from build123d import *

# Parameters (mm, degrees)
SKETCH1_W           = 16.51
SKETCH1_H           = 17.78
BOSS_EXTRUDE1_DEPTH = 1.778
FILLET1_R           = 2.54
CUT_EXTRUDE1_REACH  = 14.261
SKETCH2_R           = 0.508
SKETCH4_W           = 3.95
SKETCH4_H           = 3.95
BOSS_EXTRUDE3_DEPTH = 1.397
CUT_EXTRUDE2_REACH  = 14.261
SKETCH5_R           = 1.27


with BuildPart() as part:
    # Sketch1 → Boss-Extrude1 (new body)
    with BuildSketch(Plane(origin=(0, 0, 0), x_dir=(1, 0, 0), z_dir=(0, 1, 0))):
        Rectangle(SKETCH1_W, SKETCH1_H)
    extrude(amount=BOSS_EXTRUDE1_DEPTH)

    # Fillet1
    fillet1_edges = [part.edges().sort_by_distance(p)[0] for p in [
        (8.255, 0.889, 8.89),
        (-8.255, 0.889, 8.89),
        (-8.255, 0.889, -8.89),
        (8.255, 0.889, -8.89),
    ]]
    fillet(fillet1_edges, radius=FILLET1_R)

    # Sketch2 → Cut-Extrude1 (cut, up to next)
    with BuildSketch(Plane(origin=(0, 1.778, 0), x_dir=(1, 0, 0), z_dir=(0, 1, 0)), mode=Mode.PRIVATE) as cut_extrude1_sk1:
        with Locations(Location((-6.35, -7.112, 0), (0, 0, 270))):
            Circle(SKETCH2_R)
    cut_extrude1_tool1 = extrude(cut_extrude1_sk1.sketch, amount=-CUT_EXTRUDE1_REACH, mode=Mode.PRIVATE) & part.part
    # Sketch2 → Cut-Extrude1 (cut, up to next)
    with BuildSketch(Plane(origin=(0, 1.778, 0), x_dir=(1, 0, 0), z_dir=(0, 1, 0)), mode=Mode.PRIVATE) as cut_extrude1_sk2:
        with Locations(Location((-3.81, -7.112, 0), (0, 0, 270))):
            Circle(SKETCH2_R)
    cut_extrude1_tool2 = extrude(cut_extrude1_sk2.sketch, amount=-CUT_EXTRUDE1_REACH, mode=Mode.PRIVATE) & part.part
    # Sketch2 → Cut-Extrude1 (cut, up to next)
    with BuildSketch(Plane(origin=(0, 1.778, 0), x_dir=(1, 0, 0), z_dir=(0, 1, 0)), mode=Mode.PRIVATE) as cut_extrude1_sk3:
        with Locations(Location((-1.27, -7.112, 0), (0, 0, 270))):
            Circle(SKETCH2_R)
    cut_extrude1_tool3 = extrude(cut_extrude1_sk3.sketch, amount=-CUT_EXTRUDE1_REACH, mode=Mode.PRIVATE) & part.part
    # Sketch2 → Cut-Extrude1 (cut, up to next)
    with BuildSketch(Plane(origin=(0, 1.778, 0), x_dir=(1, 0, 0), z_dir=(0, 1, 0)), mode=Mode.PRIVATE) as cut_extrude1_sk4:
        with Locations(Location((1.27, -7.112, 0), (0, 0, 270))):
            Circle(SKETCH2_R)
    cut_extrude1_tool4 = extrude(cut_extrude1_sk4.sketch, amount=-CUT_EXTRUDE1_REACH, mode=Mode.PRIVATE) & part.part
    # Sketch2 → Cut-Extrude1 (cut, up to next)
    with BuildSketch(Plane(origin=(0, 1.778, 0), x_dir=(1, 0, 0), z_dir=(0, 1, 0)), mode=Mode.PRIVATE) as cut_extrude1_sk5:
        with Locations(Location((3.81, -7.112, 0), (0, 0, 270))):
            Circle(SKETCH2_R)
    cut_extrude1_tool5 = extrude(cut_extrude1_sk5.sketch, amount=-CUT_EXTRUDE1_REACH, mode=Mode.PRIVATE) & part.part
    # Sketch2 → Cut-Extrude1 (cut, up to next)
    with BuildSketch(Plane(origin=(0, 1.778, 0), x_dir=(1, 0, 0), z_dir=(0, 1, 0)), mode=Mode.PRIVATE) as cut_extrude1_sk6:
        with Locations(Location((6.35, -7.112, 0), (0, 0, 270))):
            Circle(SKETCH2_R)
    cut_extrude1_tool6 = extrude(cut_extrude1_sk6.sketch, amount=-CUT_EXTRUDE1_REACH, mode=Mode.PRIVATE) & part.part
    add(cut_extrude1_tool1.solids().sort_by_distance((-6.35, 1.778, 7.112))[0], mode=Mode.SUBTRACT)
    add(cut_extrude1_tool2.solids().sort_by_distance((-3.81, 1.778, 7.112))[0], mode=Mode.SUBTRACT)
    add(cut_extrude1_tool3.solids().sort_by_distance((-1.27, 1.778, 7.112))[0], mode=Mode.SUBTRACT)
    add(cut_extrude1_tool4.solids().sort_by_distance((1.27, 1.778, 7.112))[0], mode=Mode.SUBTRACT)
    add(cut_extrude1_tool5.solids().sort_by_distance((3.81, 1.778, 7.112))[0], mode=Mode.SUBTRACT)
    add(cut_extrude1_tool6.solids().sort_by_distance((6.35, 1.778, 7.112))[0], mode=Mode.SUBTRACT)

    # Sketch4 → Boss-Extrude3 (add)
    with BuildSketch(Plane(origin=(0, 0, 0), x_dir=(-1, 0, 0), z_dir=(0, -1, 0))):
        with Locations((0, 1.27)):
            Rectangle(SKETCH4_W, SKETCH4_H)
    extrude(amount=BOSS_EXTRUDE3_DEPTH)

    # Sketch5 → Cut-Extrude2 (cut, up to next)
    with BuildSketch(Plane(origin=(0, 0, 0), x_dir=(-1, 0, 0), z_dir=(0, -1, 0)), mode=Mode.PRIVATE) as cut_extrude2_sk1:
        with Locations(Location((-5.715, 6.35, 0), (0, 0, 90))):
            Circle(SKETCH5_R)
    cut_extrude2_tool1 = extrude(cut_extrude2_sk1.sketch, amount=-CUT_EXTRUDE2_REACH, mode=Mode.PRIVATE) & part.part
    # Sketch5 → Cut-Extrude2 (cut, up to next)
    with BuildSketch(Plane(origin=(0, 0, 0), x_dir=(-1, 0, 0), z_dir=(0, -1, 0)), mode=Mode.PRIVATE) as cut_extrude2_sk2:
        with Locations(Location((5.715, 6.35, 0), (0, 0, 90))):
            Circle(SKETCH5_R)
    cut_extrude2_tool2 = extrude(cut_extrude2_sk2.sketch, amount=-CUT_EXTRUDE2_REACH, mode=Mode.PRIVATE) & part.part
    add(cut_extrude2_tool1.solids().sort_by_distance((5.715, 0, -6.35))[0], mode=Mode.SUBTRACT)
    add(cut_extrude2_tool2.solids().sort_by_distance((-5.715, 0, -6.35))[0], mode=Mode.SUBTRACT)


solid = part.part
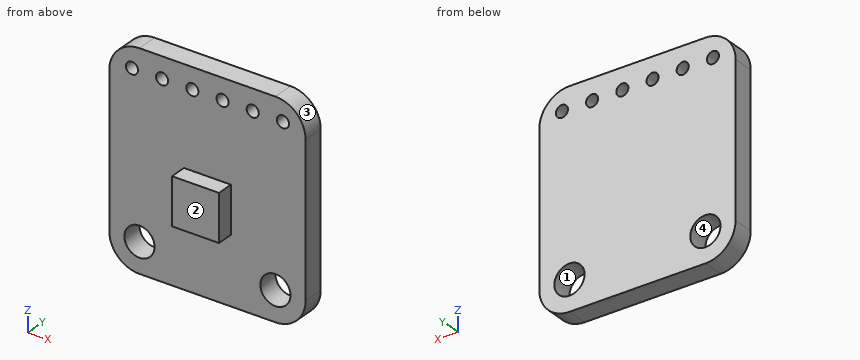
Build history of the part. All positions in model axes, mm. Face numbers are marked on the shaded views. Round coordinates to 2 decimals unless told otherwise and drop trailing zeros. Loops run counter-clockwise (first coordinate to the right, second up) from the corner with the lowest first, then second, coordinate; pieces in that order, holes last. Notation, with made-up numbers: (-18.75, 51) -> (28.25, 51) arc R15 cw to (28.25, 66) -> close; hole circle Ø10 at (-10.75, -29.5). An arc over 180 degrees is marked (long way). Use CSV: the item, a comma, the result in double quotes. Start each with the question number.
Q1. Saw through at A-A on x = -3.81. Give the cut face in (y, z).
Q2. Saw through at B-B on y = 0.4. Count the separate pieces of the cut face and the enclosed holes in it, and give its area (3 significant figures).
Q3. Mould opens along Z. For the marked faces 1, 2, 3 and 4 say: +Z half, -Z half, draft (parallel to the pull), parting line (faces both ways), or undercut.
Q4. Saw through at D-D on z = 4.25. Give the cut face in (x, y) (3 decimals).
Q5. Flat gauge pins, fed straight in: pin 1 Ø0.7 at (x, y) = (0, -0.5) entering from +Z (3 decimals); pin 2 Ø5 at (x, z) = (4, -5.5) entering from -Y; pin 3 Ø0.9 at (x, z) = (6.35, 7.112) entering from -Y (1 decimal); pin 4 Ø0.7 at (y, z) = (-0.5, -1.5) entering from +X (3 decimals). Where does each tip first touch, or does it go through?
Q6. Saw through at C-C on x = 0.5. Give the cut face in (y, z) (3 decimals).
Q7. Drill centre lines: L1, parallel to X at y = 1.25, z = -6.35 (3 decimals); L2, parallel to X at y = 1.05, z = -7; L3, parallel to Z at x = 6.5, y = 0.85. Where is each one in solid material? Low to high.
Solutions:
1,outline,"(0, -8.89) -> (1.78, -8.89) -> (1.78, 6.6) -> (0, 6.6) -> close; (0, 7.62) -> (1.78, 7.62) -> (1.78, 8.89) -> (0, 8.89) -> close"
2,separate pieces,"1"
2,enclosed holes,"8"
2,area,"273 mm^2"
3,face 1,"undercut"
3,face 2,"draft"
3,face 3,"+Z half"
3,face 4,"undercut"
4,outline,"(-8.255, 0) -> (8.255, 0) -> (8.255, 1.778) -> (-8.255, 1.778) -> close"
5,pin 1,"stops at z = 0.705"
5,pin 2,"stops at y = 0"
5,pin 3,"passes through"
5,pin 4,"stops at x = 1.975"
6,outline,"(-1.397, -3.245) -> (0, -3.245) -> (0, -8.89) -> (1.778, -8.89) -> (1.778, 8.89) -> (0, 8.89) -> (0, 0.705) -> (-1.397, 0.705) -> close"
7,L1,"x = -8.255 to -6.985, -4.445 to 4.445, 6.985 to 8.255"
7,L2,"x = -8.17 to -6.81, -4.62 to 4.62, 6.81 to 8.17"
7,L3,"z = -8.77 to -7.35, -5.35 to 6.63, 7.6 to 8.77"
